Autodesk Inventor part; units mm, degrees
ref_plane "YZ Plane" through (0, 0, 0) normal (1, 0, 0) x (0, 1, 0)
ref_plane "XZ Plane" through (0, 0, 0) normal (0, 1, 0) x (-1, 0, 0)
ref_plane "XY Plane" through (0, 0, 0) normal (0, 0, 1) x (1, 0, 0)
sketch "Sketch1" plane through (0, 0, 0) normal (0, 0, 1) x (1, 0, 0)
  line L0 (-190, 210) -> (190, 210)
  line L1 (190, 210) -> (190, -210)
  line L2 (190, -210) -> (-190, -210)
  line L3 (-190, -210) -> (-190, 210)
  point P0 (0, 0)
  point P1 (0, 210)
  point P2 (-190, 0)
  dimension "d0" = 380
  dimension "d1" = 420
extrude "Extrusion1" add sketch "Sketch1" along normal mid plane 20
sketch "Sketch5" plane through (0, 0, -10) normal (0, 0, -1) x (-1, 0, 0)
  line L0 (150, 140) -> (-190, 140)
  line L1 (-190, 140) -> (-190, -175)
  line L2 (-190, -175) -> (150, -175)
  line L3 (150, -175) -> (150, 140)
  line L4 (190, 210) -> (-190, 210)
  line L5 (-190, -210) -> (190, -210)
  line L6 (190, -210) -> (190, 210)
  point P0 (0, 0)
  dimension "d24" = 70
  dimension "d25" = 35
  dimension "d26" = 40
extrude "Extrusion5" cut sketch "Sketch5" against normal through all
sketch "Sketch6" plane through (0, 0, -10) normal (0, 0, -1) x (-1, 0, 0)
  line L0 (66.806, -190) -> (66.806, -200) construction
  line L1 (64.556, -190) -> (64.556, -200)
  line L2 (69.056, -200) -> (69.056, -190)
  arc A0 (69.056, -190) -> (64.556, -190) centre (66.806, -190) ccw
  arc A1 (64.556, -200) -> (69.056, -200) centre (66.806, -200) ccw
  line L3 (-190, -210) -> (190, -210)
  line L4 (190, -210) -> (190, 210)
  line L5 (46.806, -190) -> (46.806, -200) construction
  line L6 (44.556, -190) -> (44.556, -200)
  line L7 (49.056, -200) -> (49.056, -190)
  arc A2 (49.056, -190) -> (44.556, -190) centre (46.806, -190) ccw
  arc A3 (44.556, -200) -> (49.056, -200) centre (46.806, -200) ccw
  point P0 (0, 0)
  point P1 (66.806, -195)
  point P2 (46.806, -195)
  dimension "d30" = 15
  dimension "d32" = 123.194
  dimension "d33" = 4.5
  dimension "d34" = 10
  dimension "d36" = 20
extrude "Extrusion6" cut sketch "Sketch6" against normal through all
sketch "Sketch8" plane through (0, 0, 10) normal (0, 0, 1) x (1, 0, 0)
  circle A0 centre (-57.306, 175) radius 2
  line L0 (-79.306, 153) -> (-35.306, 153)
  line L1 (-35.306, 153) -> (-35.306, 197)
  line L2 (-35.306, 197) -> (-79.306, 197)
  line L3 (-79.306, 197) -> (-79.306, 153)
  line L4 (-79.306, 153) -> (-35.306, 197) construction
  line L5 (-35.306, 153) -> (-79.306, 197) construction
  line L6 (190, 140) -> (190, 210)
  line L7 (-190, 210) -> (-190, -210)
  point P0 (0, 0)
  point P1 (-57.306, 175)
  point P2 (190, 175)
  dimension "d45" = 44
  dimension "d67" = 132.694
extrude "Extrusion8" cut sketch "Sketch8" against normal through all contours A0 | L3 L2 L1 L0
sketch "Sketch9" plane through (0, 0, -10) normal (0, 0, -1) x (-1, 0, 0)
  line L0 (84.3, 163) -> (84.3, 147) construction
  line L1 (84.3, 147) -> (119.3, 147) construction
  line L2 (119.3, 147) -> (119.3, 163) construction
  line L3 (119.3, 163) -> (84.3, 163) construction
  line L4 (81.8, 163) -> (86.8, 163) construction
  line L5 (81.8, 160.75) -> (86.8, 160.75)
  line L6 (86.8, 165.25) -> (81.8, 165.25)
  arc A0 (81.8, 165.25) -> (81.8, 160.75) centre (81.8, 163) ccw
  arc A1 (86.8, 160.75) -> (86.8, 165.25) centre (86.8, 163) ccw
  line L7 (116.8, 163) -> (121.8, 163) construction
  line L8 (121.8, 147) -> (116.8, 147) construction
  line L9 (121.8, 149.25) -> (116.8, 149.25)
  line L10 (116.8, 144.75) -> (121.8, 144.75)
  arc A2 (121.8, 144.75) -> (121.8, 149.25) centre (121.8, 147) ccw
  arc A3 (116.8, 149.25) -> (116.8, 144.75) centre (116.8, 147) ccw
  line L11 (81.8, 147) -> (86.8, 147) construction
  line L12 (81.8, 144.75) -> (86.8, 144.75)
  line L13 (86.8, 149.25) -> (81.8, 149.25)
  arc A4 (81.8, 149.25) -> (81.8, 144.75) centre (81.8, 147) ccw
  arc A5 (86.8, 144.75) -> (86.8, 149.25) centre (86.8, 147) ccw
  circle A6 centre (121.306, 163) radius 2.75
  line L14 (190, -210) -> (190, 210)
  line L15 (190, 210) -> (-190, 210)
  line L16 (116.8, 163) -> (121.8, 163) construction
  line L17 (116.8, 165.25) -> (121.8, 165.25)
  line L18 (121.8, 160.75) -> (116.8, 160.75)
  arc A7 (116.8, 165.25) -> (116.8, 160.75) centre (116.8, 163) ccw
  arc A8 (121.8, 160.75) -> (121.8, 165.25) centre (121.8, 163) ccw
  line L19 (-190, 210) -> (190, 210)
  line L20 (-190, 140) -> (150, 140)
  point P0 (0, 0)
  dimension "d50" = 35
  dimension "d51" = 16
  dimension "d52" = 5
  dimension "d53" = 4.5
  dimension "d54" = 68.694
  dimension "d55" = 47
  dimension "d56" = 70.7
  dimension "d68" = 7
extrude "Extrusion9" cut sketch "Sketch9" against normal through all contours A0 L6 A1 L5 | A2 L10 A3 L9 | A4 L13 A5 L12 | L17 A8 L18 A6 | A6 L18 A7 L17 picked at (120.7187, 163)
pattern_linear "Rectangular Pattern1" count 2 spacing 90 along (1, 0, 0) count 2 spacing 345 along (0, -1, 0) of "Extrusion9"
sketch "Sketch10" plane through (0, 0, -10) normal (0, 0, -1) x (-1, 0, 0)
  line L0 (89.306, 200) -> (25.306, 200) construction
  line L1 (25.306, 200) -> (25.306, 183) construction
  line L2 (25.306, 183) -> (89.306, 183) construction
  line L3 (89.306, 183) -> (89.306, 200) construction
  line L4 (35.306, 197) -> (79.306, 197) construction
  line L5 (190, 210) -> (-190, 210) construction
  point P0 (0, 0)
  point P1 (57.306, 200)
  point P2 (57.306, 197)
  dimension "d69" = 64
  dimension "d70" = 10
  dimension "d71" = 17
hole "Hole1" at (-89.306, 183, -10) at (-89.306, 200, -10) at (-25.306, 200, -10) at (-25.306, 183, -10) direction (0, 0, 1) diameter 5 end through all
properties part number "0005-10-017 Batiu 2" material "Wood (Maple)"
For this review, take the finished solid that the model builds, in its own axes (mm). A direction names the side the tool comes from. Round coordinates to 2 decimals unless told otherwise and drop trailing zeros. Order: outer loops, then holes, each group sorted by start corner. A loop starts at its lowest first (then second) coordinate and runs counter-clockwise, first axis right, second up. Notation, with made-up numbers: M -3,44 L 25,44 A38 cw 25,83 Z; hole C 23.5,-7 d3. An arc over 180 degrees is marked long. Use a Markdown table: item, result. Add a question column.
Item 1: To check wall thickness, follow line 1 along X through (y, z) = (200, 5.5); line 2 along Y through (x, z) = (-39, -3.25); line 3 along Y through (x, z) = (56.5, -3.75). State the ranges of each line that lie inside material, in increasing order.
Item 2: Mouldability with a two-part tool opening along X and no side actions: class faces 4 (the flat face through (18, 140, 0)), 5 (the flat face through (-44.556, -195, 0)), 6 (the flat face through (190, -192, 0)) as released by +X, released by -X, zero draft, split by the parting line, or undercut.
Item 3: Add section B-B, the plane y = -166.5. Give the boundary of the cut face in (x, z), then the cut area to 3 significant figures.
Item 4: Insertion check: pin 1 (3 mm diameter, centred on y = -114, z = 1.5, fed in from +X). The pin has a flat end and moves straight along its axis. Give the tip position at first contact, or say it passes through.
Item 5: Add section A-A, the plane x = 39. Give the boundary of the cut face in (y, z).
Item 6: Tool access review of faces 1 (the flat face through (-150, -20, 0)), 2 (the flat face through (-58, 153, 0)), 3 (the flat face through (-45, 143, -10)): name each direction out of +Z, -Z, +X, -X, +Y, -Y from which nothing blocks a thin tool from reaching the whole face with its end or side.
Item 7: Add section C-C, the plane z = -1. State how many separate pieces and enclosed holes the cut face has, then the cut area to 3 significant figures.
Geometry results:
| question | item | result |
|---|---|---|
| 1 | line 1 | x = -190 to -91.81, -86.81 to -27.81, -22.81 to 190 |
| 1 | line 2 | y = -210 to -175, 140 to 153, 197 to 210 |
| 1 | line 3 | y = -210 to -175, 140 to 210 |
| 2 | face 4 | zero draft |
| 2 | face 5 | undercut |
| 2 | face 6 | released by +X |
| 3 | outline | M -190,-10 L -150,-10 L -150,10 L -190,10 Z |
| 3 | area | 800 mm² |
| 4 | pin 1 | stops at x = -150 |
| 5 | outline | M -210,-10 L -175,-10 L -175,10 L -210,10 Z; M 140,-10 L 210,-10 L 210,10 L 140,10 Z |
| 6 | face 1 | +Z, -Z, +X |
| 6 | face 2 | +Z, -Z |
| 6 | face 3 | -Z, +X, -X, +Y, -Y |
| 7 | separate pieces | 1 |
| 7 | enclosed holes | 23 |
| 7 | area | 49,700 mm² |
